```python
from build123d import *

# Parameters (mm, degrees)
SKETCH_1_R      = 1.5
SKETCH_1_W      = 45
SKETCH_1_H      = 25
EXTRUDE_1_DEPTH = 3
FILLET_1_R      = 2
FILLET_2_R      = 5


with BuildPart() as part:
    # 草图1 → 凸台-拉伸1 (new body)
    with BuildSketch(Plane.XY):
        Polygon((-47.5, 16), (-47.5, -16), (35.5, -16), (35.5, -11), (49.801043111, 1), (62.5, 1), (62.5, 16), (35.5, 16), align=None)
        with Locations((-29.5, 5)):
            Circle(SKETCH_1_R, mode=Mode.SUBTRACT)
        with Locations((-29.5, -5)):
            Circle(SKETCH_1_R, mode=Mode.SUBTRACT)
        with Locations((29.5, 5)):
            Circle(SKETCH_1_R, mode=Mode.SUBTRACT)
        with Locations((29.5, -5)):
            Circle(SKETCH_1_R, mode=Mode.SUBTRACT)
        with Locations((44.5, 8.5)):
            Circle(SKETCH_1_R, mode=Mode.SUBTRACT)
        with Locations((54.5, 8.5)):
            Circle(SKETCH_1_R, mode=Mode.SUBTRACT)
        with Locations((-40, 12.5)):
            Circle(SKETCH_1_R, mode=Mode.SUBTRACT)
        with Locations(Location((-40, -12.5, 0), (0, 0, 180))):
            Circle(SKETCH_1_R, mode=Mode.SUBTRACT)
        with Locations((38.5, -4)):
            Circle(SKETCH_1_R, mode=Mode.SUBTRACT)
        Rectangle(SKETCH_1_W, SKETCH_1_H, mode=Mode.SUBTRACT)
    extrude(amount=EXTRUDE_1_DEPTH)

    # 圆角1
    fillet_1_edges = [part.edges().sort_by_distance(p)[0] for p in [
        (62.5, 16, 1.5),
        (62.5, 1, 1.5),
        (49.801043111, 1, 1.5),
        (35.5, -11, 1.5),
        (35.5, -16, 1.5),
        (-47.5, -16, 1.5),
        (-47.5, 16, 1.5),
    ]]
    fillet(fillet_1_edges, radius=FILLET_1_R)

    # 圆角2
    fillet_2_edges = [part.edges().sort_by_distance(p)[0] for p in [
        (22.5, -12.5, 1.5),
        (22.5, 12.5, 1.5),
        (-22.5, 12.5, 1.5),
        (-22.5, -12.5, 1.5),
    ]]
    fillet(fillet_2_edges, radius=FILLET_2_R)


solid = part.part
```
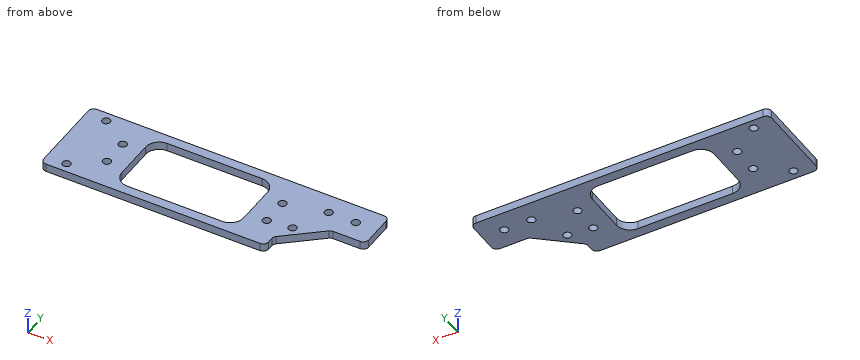
Part model, mm, in its own coordinate system. Coordinates: 2 decimals unless noted, no trailing zeros. Order: outer loops, then holes, each group sorted by start corner. A loop starts at its lowest first (then second) coordinate and runs counter-clockwise, first axis right, second up. Notation, with made-up numbers: (-32.75, 72.25) -> (-3.75, 72.25) arc R23 cw to (-3.75, 104.25) -> close; hole circle Ø6 at (45, 36). An arc over 180 degrees is marked (long way). Put each result on its own line as item: value. Start each with the question number.
(1) Band-saw the part on D-D (x = 44.5). Give the cut face in (y, z), then the cut area to 3 significant figures.
(2) Band-saw the part on C-C (z = 0.85). Count the separate pieces of the cut face and the enclosed holes in it, then the cut area to 3 significant figures.
(3) Pin check, flat tips, straight feed: pin 1 Ø1.5 at (x, z) = (54, 2) entering from -Y; pin 2 Ø0.9 at (y, z) = (-1.5, 2) entering from +X; pin 3 Ø0.6 at (y, z) = (-12.5, 1.5) entering from +X. Stop position of each tip, or through.
(4) Band-saw the part on A-A (y = 5). Give the cut face in (x, z), then the cut area to 3 significant figures.
(5) Probe line 1 along Y through (x, z) = (-40, 1); line 2 along Y through (x, z) = (-29.5, 1.85); line 3 along Y through (x, z) = (54.5, 2.35). List the from-to ranges inside material, lowest first. Write a range as [from, to].
(6) Band-saw the part on B-B (x = -40). Give the cut face in (y, z).
Determined:
1. outline: (-3.45, 0) -> (7, 0) -> (7, 3) -> (-3.45, 3) -> close; (10, 0) -> (16, 0) -> (16, 3) -> (10, 3) -> close
1. area: 49.3 mm²
2. separate pieces: 1
2. enclosed holes: 10
2. area: 1,980 mm²
3. pin 1: stops at y = 1
3. pin 2: stops at x = 47.36
3. pin 3: stops at x = 35.5
4. outline: (-47.5, 0) -> (-31, 0) -> (-31, 3) -> (-47.5, 3) -> close; (-28, 0) -> (-22.5, 0) -> (-22.5, 3) -> (-28, 3) -> close; (22.5, 0) -> (28, 0) -> (28, 3) -> (22.5, 3) -> close; (31, 0) -> (62.5, 0) -> (62.5, 3) -> (31, 3) -> close
4. area: 177 mm²
5. line 1: y = [-16, -14], [-11, 11], [14, 16]
5. line 2: y = [-16, -6.5], [-3.5, 3.5], [6.5, 16]
5. line 3: y = [1, 7], [10, 16]
6. outline: (-16, 0) -> (-14, 0) -> (-14, 3) -> (-16, 3) -> close; (-11, 0) -> (11, 0) -> (11, 3) -> (-11, 3) -> close; (14, 0) -> (16, 0) -> (16, 3) -> (14, 3) -> close
